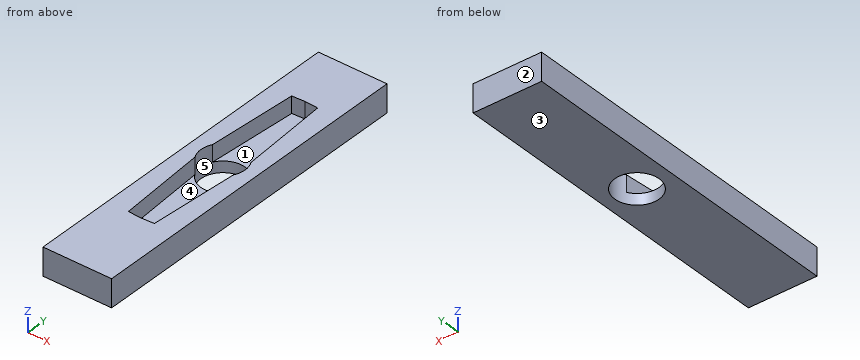
```python
from build123d import *

# Parameters (mm, degrees)
BOSS_EXTRUDE1_DEPTH = 5
CUT_EXTRUDE1_DEPTH  = 3
SKETCH4_R           = 4
CUT_EXTRUDE2_DEPTH  = 5


with BuildPart() as part:
    # Sketch1 → Boss-Extrude1 (new body)
    with BuildSketch(Plane.XY):
        Polygon((6.2, -29), (6.2, -32.59), (-6.2, -32.59), (-6.2, -29), (-6.2, 29), (6.2, 29), align=None)
    extrude(amount=-BOSS_EXTRUDE1_DEPTH)

    # Sketch2 → Cut-Extrude1 (cut)
    with BuildSketch(Plane.XY):
        Polygon((-3.613807992, 0), (-2.3482015, 18.253803872), (0, 18.387804485), (2.3482015, 18.253803872), (3.613807992, 0), (2.3482015, -18.253803872), (0, -18.387804485), (-2.3482015, -18.253803872), align=None)
    extrude(amount=-CUT_EXTRUDE1_DEPTH, mode=Mode.SUBTRACT)

    # Sketch4 → Cut-Extrude2 (cut)
    with BuildSketch(Plane.XY):
        Circle(SKETCH4_R)
    extrude(amount=-CUT_EXTRUDE2_DEPTH, mode=Mode.SUBTRACT)


solid = part.part
```
Geometry check sheet. Reference: the model listing, model coordinates, mm. Face numbers are marked on the shaded views. A direction names the side the tool comes from. Coordinates: 2 decimals unless noted, no trailing zeros. Order: outer loops, then holes, each group sorted by start corner. A loop starts at its lowest first (then second) coordinate and runs counter-clockwise, first axis right, second up.
Q1. Sectioned sample at C-C on z = -3.65. Record the cut outline in (x, y).
Reply:
outline: (-6.2, -32.59) - (6.2, -32.59) - (6.2, 29) - (-6.2, 29) - close; hole circle Ø8 at (0, 0)
Q2. Depth check by flat-ended pin: pin 1 Ø2 at (x, y) = (0.5, 7.5) entering from +Z. Enter the tip coordinate at first touch or a pass-through.
Reply:
pin 1: stops at z = -3
Q3. Thickness scan on probe 1 along X at (y, z) = (0, -1.8); probe 2 along Y at (x, z) = (0, -2.2); probe 3 along X at (y, z) = (-2, -1.4). Record the ranges inside material, lowest first.
Reply:
probe 1: x = -6.2 to -4, 4 to 6.2
probe 2: y = -32.59 to -18.39, 18.39 to 29
probe 3: x = -6.2 to -3.48, 3.48 to 6.2
Q4. Sectioned sample at D-D on y = 15.5. Record the cut outline in (x, z).
Reply:
outline: (-6.2, -5) - (6.2, -5) - (6.2, 0) - (2.54, 0) - (2.54, -3) - (-2.54, -3) - (-2.54, 0) - (-6.2, 0) - close
Q5. Sectioned sample at B-B on x = 1.25. Record the cut outline in (y, z).
Reply:
outline: (-32.59, -5) - (-3.8, -5) - (-3.8, -3) - (-18.32, -3) - (-18.32, 0) - (-32.59, 0) - close; (3.8, -5) - (29, -5) - (29, 0) - (18.32, 0) - (18.32, -3) - (3.8, -3) - close
Q6. Sectioned sample at A-A on y = 0. Record the cut outline in (x, z).
Reply:
outline: (-6.2, -5) - (-4, -5) - (-4, 0) - (-6.2, 0) - close; (4, -5) - (6.2, -5) - (6.2, 0) - (4, 0) - close
Q7. Draft check along Y on the marked faces 1, 2 and 3. Enter one of: released by +Y, released by -Y, zero draft, split by the parting line, or undercut.
Reply:
face 1: undercut
face 2: released by +Y
face 3: zero draft
Q8. Tool access check on the marked faces 4 and 5. Record the directions out of +Z, -Z, +X, -X, +Y, -Y that give a thin tool (end or side, any length) a straight path to the whole face; none if there is none.
Reply:
face 4: +Z
face 5: +Z, -Z
